from build123d import *

# Parameters (mm, degrees)
SKETCH_1_R          = 18.5
EXTRUDE_3_DEPTH     = 23
SKETCH_3_R          = 16.5
EXTRUDE_4_DEPTH     = 23
SKETCH_4_R          = 6
EXTRUDE_5_DEPTH     = 6
SKETCH_6_R          = 3
EXTRUDE_6_DEPTH     = 12
SKETCH_7_R          = 2
EXTRUDE_7_DEPTH     = 2
SKETCH_8_W          = 3
SKETCH_8_H          = 1
EXTRUDE_8_DEPTH     = 7
SKETCH_9_R          = 16.5
EXTRUDE_9_DEPTH     = 2
SKETCH_10_W         = 4.5
SKETCH_10_H         = 12
EXTRUDE_10_DEPTH    = 5
FILLET_1_R          = 1
SKETCH_11_R         = 8
EXTRUDE_11_DEPTH    = 4
SKETCH_12_R         = 1.6
CUT_EXTRUDE_1_DEPTH = 2


with BuildPart() as part:
    # 草图1 → 凸台-拉伸3 (new body)
    with BuildSketch(Plane.XY):
        Circle(SKETCH_1_R)
    extrude(amount=EXTRUDE_3_DEPTH)

    # 草图3 → 凸台-拉伸4 (add)
    with BuildSketch(Plane.XY.offset(23)):
        Circle(SKETCH_3_R)
    extrude(amount=EXTRUDE_4_DEPTH)

    # 草图4 → 凸台-拉伸5 (add)
    with BuildSketch(Plane(origin=(0, 0, 0), x_dir=(-1, 0, 0), z_dir=(0, 0, -1))):
        with Locations(Location((0, 7, 0), (0, 0, 180))):
            Circle(SKETCH_4_R)
    extrude(amount=EXTRUDE_5_DEPTH)

    # 草图6 → 凸台-拉伸6 (add)
    with BuildSketch(Plane(origin=(0, 0, -6), x_dir=(-1, 0, 0), z_dir=(0, 0, -1))):
        with Locations((0, 7)):
            Circle(SKETCH_6_R)
    extrude(amount=EXTRUDE_6_DEPTH)

    # 草图7 → 凸台-拉伸7 (add)
    with BuildSketch(Plane.XY.offset(46)):
        Circle(SKETCH_7_R)
    extrude(amount=EXTRUDE_7_DEPTH)

    # 草图8 → 凸台-拉伸8 (add)
    with BuildSketch(Plane.XY.offset(46)):
        with Locations((0, -12)):
            Rectangle(SKETCH_8_W, SKETCH_8_H)
        with Locations((0.066509227, 12)):
            Rectangle(SKETCH_8_W, SKETCH_8_H)
    extrude(amount=EXTRUDE_8_DEPTH)

    # 草图9 → 凸台-拉伸9 (add)
    with BuildSketch(Plane.XY.offset(48)):
        Circle(SKETCH_9_R)
    extrude(amount=EXTRUDE_9_DEPTH)

    # 草图10 → 凸台-拉伸10 (add)
    with BuildSketch(Plane.XY.offset(50)):
        with Locations((15, 0)):
            Rectangle(SKETCH_10_W, SKETCH_10_H)
    extrude(amount=EXTRUDE_10_DEPTH)

    # 圆角1
    fillet_1_edges = [part.edges().sort_by_distance(p)[0] for p in [
        (1.566509227, 12, 53),
        (-1.433490773, 12, 53),
        (1.5, -12, 53),
        (-1.5, -12, 53),
    ]]
    fillet(fillet_1_edges, radius=FILLET_1_R)

    # 草图11 → 凸台-拉伸11 (add)
    with BuildSketch(Plane.XY.offset(50)):
        Circle(SKETCH_11_R)
    extrude(amount=EXTRUDE_11_DEPTH)

    # 草图12 → 切除-拉伸1 (cut)
    with BuildSketch(Plane(origin=(0, 0, 0), x_dir=(-1, 0, 0), z_dir=(0, 0, -1))):
        with Locations((15.5, 0)):
            Circle(SKETCH_12_R)
        with Locations((7.75, -13.423393759)):
            Circle(SKETCH_12_R)
        with Locations((-7.75, -13.423393759)):
            Circle(SKETCH_12_R)
        with Locations((-15.5, 0)):
            Circle(SKETCH_12_R)
        with Locations((-7.75, 13.423393759)):
            Circle(SKETCH_12_R)
        with Locations((7.75, 13.423393759)):
            Circle(SKETCH_12_R)
    extrude(amount=-CUT_EXTRUDE_1_DEPTH, mode=Mode.SUBTRACT)


solid = part.part
Can you work these out from the model? Positions are in its coordinate system, mm. A direction names the side the tool comes from. Round coordinates to 2 decimals unless told otherwise and drop trailing zeros. Write each loop counter-clockwise with the first axis right and the second up, starting at its lowest first coordinate (ties: lowest second). Pieces come first, ordered by that corner, then holes. Notation, with made-up numbers: M 44.5,-14 L 86.5,-14 A20 cw 86.5,4 Z; hole C 29.5,-32.75 d7. An arc over 180 degrees is marked long. Use a Markdown table: item, result.
Item 1: I want a section at A-A (x = -11.5). List the corners of the cut face in (y, z) for me, and give its area (3 significant figures).
Found:
| item | result |
|---|---|
| outline | M -14.49,0 L 14.49,0 L 14.49,23 L 11.83,23 L 11.83,46 L -11.83,46 L -11.83,23 L -14.49,23 Z; M -11.83,48 L 11.83,48 L 11.83,50 L -11.83,50 Z |
| area | 1,260 mm2 |
Item 2: If I drill on line 1 along Z through (x, y) = (15, 4); line 2 along Z through (x, y) = (9, 10); line 3 along Y through (x, z) = (7.75, 1.15), over which ranges is the centre line in solid material (lowest first)? Write a range as [from, to].
Found:
| item | result |
|---|---|
| line 1 | z = [0, 46], [48, 55] |
| line 2 | z = [0, 46], [48, 50] |
| line 3 | y = [-16.8, -15.02], [-11.82, 11.82], [15.02, 16.8] |
Item 3: I want a section at D-D (z = 36). List the corners of the cut face in (x, y) for me, and give its area (3 significant figures).
Found:
| item | result |
|---|---|
| outline | C 0,0 d33 |
| area | 855 mm2 |
Item 4: For pin 1 Ø1 at (x, y) = (-8, -14) entering from -Z; pin 2 Ø5 at (x, y) = (7.5, 9) entering from -Z; pin 3 Ø1.5 at (y, z) = (-7.5, 30) entering from -X, each with a flat end and sliding along its axis, tell me the tip position at first contact or that it passes through.
Found:
| item | result |
|---|---|
| pin 1 | stops at z = 2 |
| pin 2 | stops at z = -6 |
| pin 3 | stops at x = -15.06 |
Item 5: I want a section at B-B (y = 7). List the corners of the cut face in (x, z) for me, and give its area (3 significant figures).
Found:
| item | result |
|---|---|
| outline | M -17.12,0 L -6,0 L -6,-6 L -3,-6 L -3,-18 L 3,-18 L 3,-6 L 6,-6 L 6,0 L 17.12,0 L 17.12,23 L 14.94,23 L 14.94,46 L -14.94,46 L -14.94,23 L -17.12,23 Z; M -14.94,48 L 14.94,48 L 14.94,50 L 3.87,50 L 3.87,54 L -3.87,54 L -3.87,50 L -14.94,50 Z |
| area | 1,710 mm2 |
Item 6: We'd pull the mould along X, two halves only. Please class faces 1 (the face through (17.25, 0, 52)), 2 (the face through (12.75, 0, 52)), 3 (the face through (0, -12.5, 47)): released by +X, released by -X, zero draft, split by the parting line, or undercut.
Found:
| item | result |
|---|---|
| face 1 | released by +X |
| face 2 | undercut |
| face 3 | zero draft |
Item 7: Which directions (+Z, -Z, +X, -X, +Y, -Y) give clear straight access to the entire face, cutting with the end or side of a thin tool? Please do faces 4 (the face through (16, 0, 2)), 5 (the face through (0, 0, 54)), 6 (the face through (-1.73, -7.81, 51.97)), 7 (the face through (15, 6, 52)).
Found:
| item | result |
|---|---|
| face 4 | -Z |
| face 5 | +Z, -X, +Y, -Y |
| face 6 | +Z |
| face 7 | +Z, +X, +Y |
